Study the drawing (mm; zero at the part's minimum x, y, z) and answer. A direction names the side the tool comes from. Round coordinates to 2 decimals unless told otherwise and drop trailing zeros. Write each loop counter-clockwise with the first axis right and the second up, starting at its lowest first coordinate (ties: lowest second). Pieces come first, ordered by that corner, then holes.
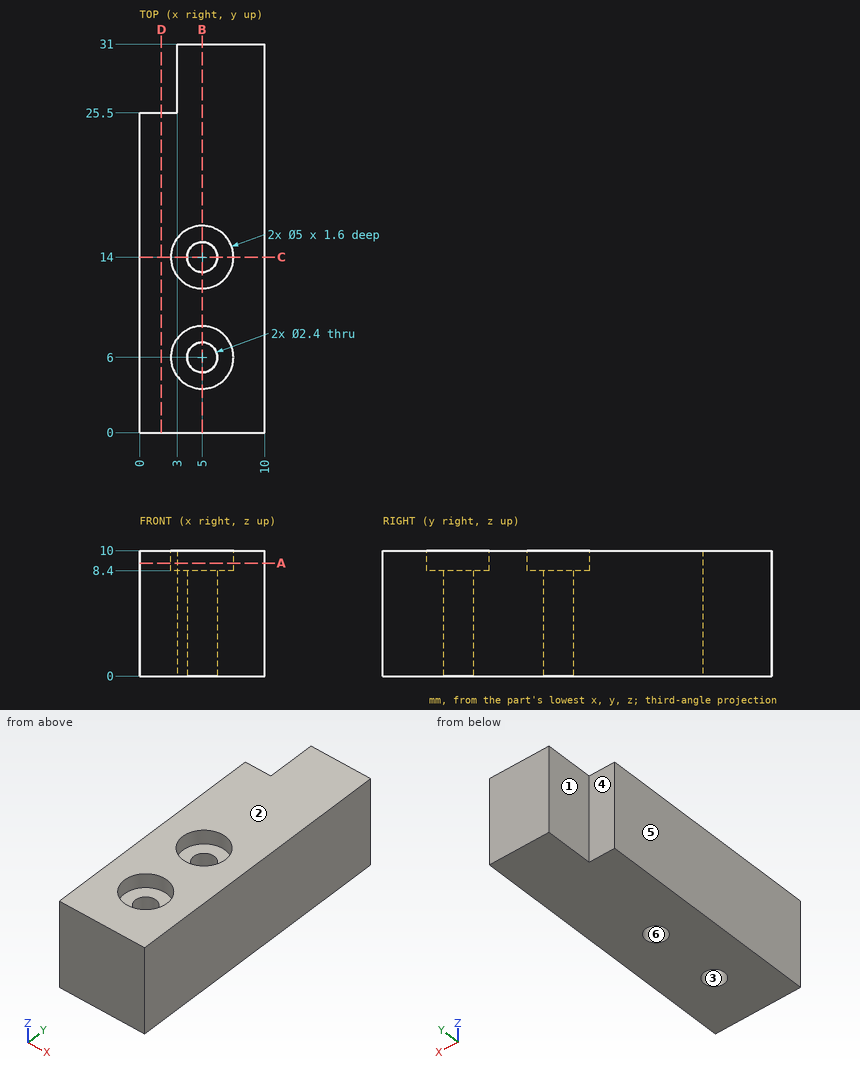
1. A tool of negligible diameter and unlimited length cuts with its end or side. For the marked faces 1 and 2, from which of +Z, -Z, +X, -X, +Y, -Y can it reach the whole face along a straight path? Write none if from no direction.
Geometry says:
face 1: +Z, -Z, -X, +Y
face 2: +Z, +X, -X, +Y, -Y
2. Straight lines are drawn through the part: line 1 along Y through (x, z) = (5, 4); line 2 along Y through (x, z) = (5, 9); line 3 along X through (y, z) = (6, 2.5). For each, find the intervals that lie inside material, in ascending order.
Geometry says:
line 1: y = 0 to 4.8, 7.2 to 12.8, 15.2 to 31
line 2: y = 0 to 3.5, 8.5 to 11.5, 16.5 to 31
line 3: x = 0 to 3.8, 6.2 to 10
3. For a pull along Y with two mould halves and no side action, classify the marked faces 3, 4, 5 and 6 as released by +Y, released by -Y, zero draft, split by the parting line, or undercut.
Geometry says:
face 3: undercut
face 4: released by +Y
face 5: zero draft
face 6: undercut
4. Section C-C on y = 14 is taken. Determine the outline of the cut face in (x, z).
Geometry says:
outline: (0, 0) - (3.8, 0) - (3.8, 8.4) - (2.5, 8.4) - (2.5, 10) - (0, 10) - close; (6.2, 0) - (10, 0) - (10, 10) - (7.5, 10) - (7.5, 8.4) - (6.2, 8.4) - close
5. Section D-D on x = 1.75 is taken. Determine the outline of the cut face in (y, z).
Geometry says:
outline: (0, 0) - (25.5, 0) - (25.5, 10) - (0, 10) - close
6. Given pin 1 (3 mm diameter, centred on y = 29, z = 6.5, fed in from -X); pin 2 (1.5 mm diameter, centred on x = 1.5, z = 6, fed in from +Y); pin 3 (1.5 mm diameter, centred on x = 5.5, y = 6.5, fed in from +Z); pin 4 (1.9 mm diameter, centred on x = 5, y = 14, fed in from +Z), each flat-ended and moving along its own axis, determine where each tip first touches the part or whether it passes through.
Geometry says:
pin 1: stops at x = 3
pin 2: stops at y = 25.5
pin 3: stops at z = 8.4
pin 4: passes through
7. Section B-B on x = 5 is taken. Determine the outline of the cut face in (y, z), plus the area to 3 significant figures.
Geometry says:
outline: (0, 0) - (4.8, 0) - (4.8, 8.4) - (3.5, 8.4) - (3.5, 10) - (0, 10) - close; (7.2, 0) - (12.8, 0) - (12.8, 8.4) - (11.5, 8.4) - (11.5, 10) - (8.5, 10) - (8.5, 8.4) - (7.2, 8.4) - close; (15.2, 0) - (31, 0) - (31, 10) - (16.5, 10) - (16.5, 8.4) - (15.2, 8.4) - close
area: 254 mm2
8. Section A-A on z = 9 is taken. Determine the outline of the cut face in (x, y), plus the area to 3 significant figures.
Geometry says:
outline: (0, 0) - (10, 0) - (10, 31) - (3, 31) - (3, 25.5) - (0, 25.5) - close; hole circle Ø5 at (5, 6); hole circle Ø5 at (5, 14)
area: 254 mm2
